```python
from build123d import *

# Parameters (mm, degrees)
SKETCH2_R           = 14
SKETCH2_R_2         = 8
BOSS_EXTRUDE1_DEPTH = 56
SKETCH4_R           = 14
SKETCH4_R_2         = 8
BOSS_EXTRUDE2_DEPTH = 28


with BuildPart() as part:
    # Sketch2 → Boss-Extrude1 (new body)
    with BuildSketch(Plane(origin=(0, 0, 0), x_dir=(0, 1, 0), z_dir=(0, 0, 1))):
        with Locations(Location((0, 0, 0), (0, 0, 270))):
            Circle(SKETCH2_R)
        with Locations(Location((0, 0, 0), (0, 0, 270))):
            Circle(SKETCH2_R_2, mode=Mode.SUBTRACT)
    extrude(amount=BOSS_EXTRUDE1_DEPTH)

    # Sketch4 → Boss-Extrude2 (add, symmetric)
    with BuildSketch(Plane.YZ):
        with Locations(Location((24, 28.13266563, 0), (0, 0, 270))):
            Circle(SKETCH4_R)
        with Locations(Location((24, 28.13266563, 0), (0, 0, 270))):
            Circle(SKETCH4_R_2, mode=Mode.SUBTRACT)
    extrude(amount=BOSS_EXTRUDE2_DEPTH, both=True)


solid = part.part
```
Verification items for the finished model (mm, model axes). Give positions to 0.01 mm unless a question says otherwise; leave off trailing zeros. Order: outer loops, then holes, each group sorted by start corner. A loop starts at its lowest first (then second) coordinate and runs counter-clockwise, first axis right, second up. Notation, with made-up numbers: (-12, 89) -> (31, 89) arc R9 ccw to (31, 98) -> close; hole circle Ø5 at (37, 27.25). An arc over 180 degrees is marked (long way). Use a Markdown table: item, result.
1) Mould release check, pull along X, two halves, no side actions. Record for faces 1 (the cylindrical face through (-1.73, -7.81, 27.61)), 2 (the cylindrical face through (-0.4, 26.4, 20.5)), 3 (the flat face through (28, 18, 22)): pulls with the +X half, pulls with the -X half, needs draft (parallel to the pull), parting line crosses it, or undercut.
Results:
| item | result |
|---|---|
| face 1 | undercut |
| face 2 | needs draft |
| face 3 | pulls with the +X half |
2) Section check C-C, the plane z = 34.5. Record the boundary of the cut face in (x, y), then the cut area to 3 significant figures.
Results:
| item | result |
|---|---|
| outline | (-28, 11.53) -> (-7.94, 11.53) arc R14 ccw (long way) to (7.94, 11.53) -> (28, 11.53) -> (28, 19.16) -> (-28, 19.16) -> close; (-28, 28.84) -> (28, 28.84) -> (28, 36.47) -> (-28, 36.47) -> close; hole circle Ø16 at (0, 0) |
| area | 1,240 mm² |
3) Section check A-A, the plane y = 24. Record the boundary of the cut face in (x, z).
Results:
| item | result |
|---|---|
| outline | (-28, 14.13) -> (28, 14.13) -> (28, 20.13) -> (-28, 20.13) -> close; (-28, 36.13) -> (28, 36.13) -> (28, 42.13) -> (-28, 42.13) -> close |
4) Section check B-B, the plane x = -4. Record the boundary of the cut face in (y, z), then the cut area to 3 significant figures.
Results:
| item | result |
|---|---|
| outline | (-13.42, 0) -> (-6.93, 0) -> (-6.93, 56) -> (-13.42, 56) -> close; (6.93, 0) -> (13.42, 0) -> (13.42, 18.97) arc R14 ccw (long way) to (13.42, 37.3) -> (13.42, 56) -> (6.93, 56) -> close; hole circle Ø16 at (24, 28.13) |
| area | 1,100 mm² |
5) Depth check by flat-ended pin: pin 1 Ø14.5 at (y, z) = (24, 28.13) entering from +X; pin 2 Ø6 at (x, z) = (-6, 46) entering from -Y; pin 3 Ø8 at (x, y) = (21.5, 31.5) entering from -Z; pin 4 Ø2 at (x, z) = (-16.5, 26.5) entering from -Y. Enter the tip coordinate at first touch or a pass-through.
Results:
| item | result |
|---|---|
| pin 1 | through |
| pin 2 | y = -13.67 |
| pin 3 | z = 14.58 |
| pin 4 | y = 10.01 |
6) Material ranges on probe 1 along Y at (x, z) = (-12.5, 31.5); probe 2 along Y at (x, z) = (0, 32); probe 3 along Y at (x, z) = (-0.5, 13), recorded low to high.
Results:
| item | result |
|---|---|
| probe 1 | -6.3 to 6.3, 10.41 to 16.74, 31.26 to 37.59 |
| probe 2 | -14 to -8, 8 to 17, 31 to 37.46 |
| probe 3 | -13.99 to -7.98, 7.98 to 13.99 |
7) Section check D-D, the plane x = -23. Record the boundary of the cut face in (y, z), then the cut area to 3 significant figures.
Results:
| item | result |
|---|---|
| outline | circle Ø28 at (24, 28.13); hole circle Ø16 at (24, 28.13) |
| area | 415 mm² |
